from build123d import *

# Parameters (mm, degrees)
F1_DEPTH = 80
F2_R     = 3
F3_R     = 3


with BuildPart() as f1:
    # F0 (on Top) → F1 (new body)
    with BuildSketch(Plane.XY):
        with BuildLine():
            Line((-40, 7), (-40, -41))
            Line((-40, -41), (40, -41))
            Line((40, -41), (40, 41))
            ThreePointArc((40, 41), (35.6846584384, 48.6846584384), (26.8768943744, 49))
            ThreePointArc((26.8768943744, 49), (21.6884164325, 37.9773734121), (31, 30.1216104501))
            ThreePointArc((31, 30.1216104501), (32.9083754305, 28.1237103179), (31, 26.1258101857))
            add(Edge.make_bspline(
                [(31, 26.1258101857), (29.1383194506, 2.2108836058), (30.9167526541, -31.2253562681), (8.8170867264, -33.1853542307), (0, -33.4819146159)],
                knots=[0, 0, 0, 0, 0.6000833432, 1, 1, 1, 1], degree=3))
            ThreePointArc((0, -33.4819146159), (-8.7763698001, -32.5596158188), (-16.9671031431, -29.2752301466))
            add(Edge.make_bspline(
                [(-16.9671031431, -29.2752301466), (-14.901822055, -25.8906310448), (-16.1565216247, -25.0924466589), (-17.4112211944, -24.2942622731), (-19.4985771018, -27.664818351)],
                knots=[4.7144665779, 4.7144665779, 4.7144665779, 6.2764659366, 6.2764659366, 7.8384652954, 7.8384652954, 7.8384652954], degree=2, weights=[1, 0.710210129, 1, 0.710210129, 1]))
            ThreePointArc((-19.4985771018, -27.664818351), (-24.3581566231, -23.452844128), (-28.2774287922, -18.3542614188))
            add(Edge.make_bspline(
                [(-28.2774287922, -18.3542614188), (-25.5565793832, -15.5150943204), (-26.3141793997, -14.1455346477), (-27.0717794162, -12.7759749751), (-29.8082391869, -15.5869222722)],
                knots=[1.4456697136, 1.4456697136, 1.4456697136, 3.0061633493, 3.0061633493, 4.566656985, 4.566656985, 4.566656985], degree=2, weights=[1, 0.7107399344, 1, 0.7107399344, 1]))
            ThreePointArc((-29.8082391869, -15.5869222722), (-32.3036744342, -8.4866885025), (-33.0717967697, -1))
            ThreePointArc((-33.0717967697, -1), (-34.7084973779, 4.582575695), (-40, 7))
        make_face()
    extrude(amount=F1_DEPTH)

    # F2
    f2_edges = [f1.edges().sort_by_distance(p)[0] for p in [
        (-40, 7, 40),
    ]]
    fillet(f2_edges, radius=F2_R)

    # F3
    f3_edges = [f1.edges().sort_by_distance(p)[0] for p in [
        (31, 26.12581, 40),
    ]]
    fillet(f3_edges, radius=F3_R)


solid = f1.part
Can you work these out from the model? Positions are in its coordinate system, mm. A direction names the side the tool comes from. Give positions to 0.01 mm unless a question says otherwise; leave off trailing zeros. Write each loop counter-clockwise with the first axis right and the second up, starting at its lowest first coordinate (ties: lowest second). Pieces come first, ordered by that corner, then holes. Notation, with made-up numbers: M 60,-9.5 L 93,-9.5 A8 ccw 93,3.5 Z; hole C 32,-9.5 d4. An arc over 180 degrees is marked long. Answer in a Markdown table with one row per item. Add a question column.
Item 1: We'd pull the mould along X, two halves only. Please class faces 1 (the cylindrical face through (-32.28, -8.59, 39.44)), 2 (the cylindrical face through (-24.296, -23.518, 39.44)), 3 (the cylindrical face through (21.65, 38.16, 39.44)), 4 (the flat face through (29, -9, 80)): released by +X, released by -X, zero draft, split by the parting line, or undercut.
Item 2: Imagine slicing it at A-A, the plane x = -12. Write out the boundary of the cut face in (y, z), plus the area to 3 significant figures.
Item 3: Please list where these lines run through material, in increasing order: L1, parallel to X at y = -23, z = 45; L2, parallel to Y at x = -16.5, z = 69; L3, parallel to X at y = -31, z = 69.
Item 4: On a 3-axis mill with a long thin cutter (end or side, diameter ignored), from which of +Z, -Z, +X, -X, +Y, -Y can I reach the whole of each face in a straight line? I mean faces 5 (the flat face through (29, -9, 0)), 6 (the cylindrical face through (-33.28, 1.96, 39.44)). Say none if no direction works.
Item 5: For pin 1 Ø5 at (x, z) = (7.5, 60.5) entering from +Y; pin 2 Ø12 at (y, z) = (39.5, 71) entering from -X; pin 3 Ø8 at (x, z) = (-26, 65.5) entering from +Y, each with a flat end and sliding along its axis, tell me the tip position at first contact or that it passes through.
Evaluation:
| question | item | result |
|---|---|---|
| 1 | face 1 | undercut |
| 1 | face 2 | undercut |
| 1 | face 3 | released by -X |
| 1 | face 4 | zero draft |
| 2 | outline | M -41,0 L -31.58,0 L -31.58,80 L -41,80 Z |
| 2 | area | 754 mm² |
| 3 | L1 | x = -40 to -24.78, 25.02 to 40 |
| 3 | L2 | y = -41 to -29.54, -28.42 to -25 |
| 3 | L3 | x = -40 to -13.48, 16.26 to 40 |
| 4 | face 5 | -Z, +X, -X, +Y, -Y |
| 4 | face 6 | +Z, -Z |
| 5 | pin 1 | stops at y = -32.66 |
| 5 | pin 2 | stops at x = 21.46 |
| 5 | pin 3 | stops at y = -13.83 |
